For this review, take the finished solid that the model builds, in its own axes (mm). A direction names the side the tool comes from. Give positions to 0.01 mm unless a question says otherwise; leave off trailing zeros. Order: outer loops, then holes, each group sorted by start corner. A loop starts at its lowest first (then second) coordinate and runs counter-clockwise, first axis right, second up. Notation, with made-up numbers: (28, 10) -> (87, 10) arc R24 cw to (87, 26) -> close; hole circle Ø4 at (21, 82). An arc over 180 degrees is marked (long way). Return JSON: item names as keys, results as strings. Group by question number.
1) Add section C-C (x = -45.5). Give the boundary of the cut face in (y, z).
2) For faces 5 (the face through (-36, -85.934, 1)), 6 (the face through (-147.27, -78.74, 1.48)), list the 3-axis set-ups (+Z, -Z, +X, -X, +Y, -Y) from which the entire face can be reached by the end or side of a thin tool; tool diameter is ignored.
3) To check wall thickness, follow line 1 along X through (y, z) = (-3, 1.4); line 2 along Y through (x, z) = (-24.5, 2.55); line 3 along X through (y, z) = (-72.5, 2.25). State the ranges of each line that lie inside material, in increasing order.
4) Add section B-B (x = -99). Give the boundary of the cut face in (y, z), then the cut area to 3 significant figures.
5) Add section A-A (z = 2.3). State how many separate pieces and enclosed holes the cut face has, then the cut area to 3 significant figures.
6) Insertion check: P1, Ø0.9, axis at x = -31, z = 1.5, coming from the -Y side. The pin has a flat end and moves straight along its axis. Give the tip position at first contact, or say it passes through.
7) The part is to be moulded in two halves that separate along X. For faces 1 (the face through (-144.545, -22.291, 1.479)), 2 (the face through (-86, -42, 3)), 3 (the face through (-157.241, 3.145, 1.479)), 4 (the face through (-111.996, -1.608, 1.479)), say which applies: released by +X, released by -X, zero draft, split by the parting line, or undercut.
from build123d import *

# Parameters (mm, degrees)
ESQUISSE1_R        = 1.6
BOSS_EXTRU_1_DEPTH = 3


with BuildPart() as part:
    # Esquisse1 → Boss.-Extru.1 (new body)
    with BuildSketch(Plane.XY):
        Polygon((-15.693595538, 5.608560861), (-96.367147031, 5.364168479), (-103.365175584, 5.364168479), (-119.344550333, 5.364168479), (-140.021777649, 5.320852512), (-155.064772313, 5.320852512), (-159.478985875, 0.90663895), (-159.478985875, -3.429484403), (-159.478985875, -70.574320891), (-133.100653393, -116.486520024), (-127.076613358, -118.11178196), (-105.412894174, -105.642711064), (-64.97062335, -99.631001274), (-54.971738012, -85.933633781), (-15.772854297, -85.933633781), (-11.339106961, -81.196072129), (-11.339106961, 1.267243786), align=None)
        with Locations((-18.339106961, -1.341926987)):
            Circle(ESQUISSE1_R, mode=Mode.SUBTRACT)
        with Locations((-110.397084988, -1.678365923)):
            Circle(ESQUISSE1_R, mode=Mode.SUBTRACT)
        with Locations((-18.339106961, -78.933633781)):
            Circle(ESQUISSE1_R, mode=Mode.SUBTRACT)
        with Locations((-68.897334865, -93.137788223)):
            Circle(ESQUISSE1_R, mode=Mode.SUBTRACT)
        with Locations((-128.322250168, -110.752044388)):
            Circle(ESQUISSE1_R, mode=Mode.SUBTRACT)
        with Locations((-146.0923789, -79.822656053)):
            Circle(ESQUISSE1_R, mode=Mode.SUBTRACT)
        with Locations((-146.02282508, -1.677868186)):
            Circle(ESQUISSE1_R, mode=Mode.SUBTRACT)
        with Locations((-146.02282508, -21.677868186)):
            Circle(ESQUISSE1_R, mode=Mode.SUBTRACT)
    extrude(amount=BOSS_EXTRU_1_DEPTH)


solid = part.part
Evaluation:
{
 "1": {"outline": "(-85.93, 0) -> (5.52, 0) -> (5.52, 3) -> (-85.93, 3) -> close"},
 "2": {"face 5": "+Z, -Z, +X, -Y", "face 6": "+Z, -Z"},
 "3": {"line 1": "-159.48 to -146.92, -145.12 to -111.3, -109.5 to -11.34", "line 2": "-85.93 to 5.58", "line 3": "-158.37 to -11.34"},
 "4": {"outline": "(-104.69, 0) -> (5.36, 0) -> (5.36, 3) -> (-104.69, 3) -> close", "area": "330 mm^2"},
 "5": {"separate pieces": "1", "enclosed holes": "8", "area": "15,100 mm^2"},
 "6": {"P1": "y = -85.93"},
 "7": {"face 1": "undercut", "face 2": "zero draft", "face 3": "released by -X", "face 4": "undercut"}
}
